```python
from build123d import *

# Parameters (mm, degrees)
MODEL_R                 = 1.5
SALIENTE_EXTRUIR1_DEPTH = 3


with BuildPart() as part:
    # Model → Saliente-Extruir1 (new body)
    with BuildSketch(Plane.XY):
        with BuildLine():
            Line((348.865624859, 201.955720999), (341.183644344, 209.637701515))
            ThreePointArc((341.183644344, 209.637701515), (334.819683313, 209.637701515), (334.819683313, 203.273740484))
            Line((334.819683313, 203.273740484), (343.819683313, 194.273740484))
            ThreePointArc((343.819683313, 194.273740484), (344.50159778, 193.714107744), (345.279588383, 193.298263103))
            Line((345.279588383, 193.298263103), (372.279588383, 175.298263103))
            ThreePointArc((372.279588383, 175.298263103), (373.123757379, 175.042187237), (374.001663828, 174.955720999))
            Line((374.001663828, 174.955720999), (383.001663828, 174.955720999))
            ThreePointArc((383.001663828, 174.955720999), (387.501663828, 179.455720999), (383.001663828, 183.955720999))
            Line((383.001663828, 183.955720999), (375.865624859, 183.955720999))
            Line((375.865624859, 183.955720999), (369.501663828, 190.31968203))
            Line((369.501663828, 190.31968203), (369.501663828, 197.455720999))
            ThreePointArc((369.501663828, 197.455720999), (368.183644344, 200.637701515), (365.001663828, 201.955720999))
            Line((365.001663828, 201.955720999), (348.865624859, 201.955720999))
        make_face()
        with Locations((347.001663829, 197.455720999)):
            Circle(MODEL_R, mode=Mode.SUBTRACT)
        with Locations((338.001663828, 206.455720999)):
            Circle(MODEL_R, mode=Mode.SUBTRACT)
        with Locations((365.001663828, 188.455720999)):
            Circle(MODEL_R, mode=Mode.SUBTRACT)
        with Locations((356.001663828, 197.455720999)):
            Circle(MODEL_R, mode=Mode.SUBTRACT)
        with Locations((383.001663828, 179.455720999)):
            Circle(MODEL_R, mode=Mode.SUBTRACT)
        with Locations((365.001663828, 197.455720999)):
            Circle(MODEL_R, mode=Mode.SUBTRACT)
    extrude(amount=SALIENTE_EXTRUIR1_DEPTH)


solid = part.part
```
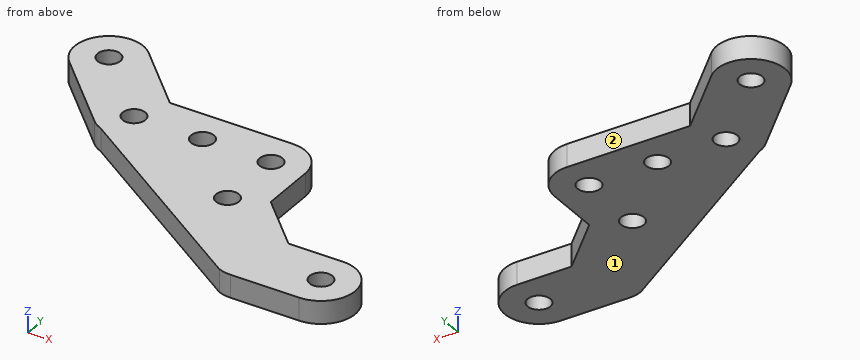
The model under review builds one solid part; all positions refer to its coordinate system, in mm. Face numbers are marked on the shaded views. A direction names the side the tool comes from. Coordinates: 2 decimals unless noted, no trailing zeros. Order: outer loops, then holes, each group sorted by start corner. A loop starts at its lowest first (then second) coordinate and runs counter-clockwise, first axis right, second up. Notation, with made-up numbers: (63.5, 47.5) -> (114.5, 47.5) arc R19 ccw to (114.5, 65.5) -> close; hole circle Ø9 at (-31.5, 51). An arc over 180 degrees is marked (long way). Answer in a Markdown table with one row per item. Add a question column.
Item 1: Clearance check with flat-ended pins moving along their axes: pin 1 (0.9 mm diameter, centred on y = 193, z = 1, fed in from +X); pin 2 (1.5 mm diameter, centred on x = 368, z = 1, fed in from -Y); pin 3 (0.9 mm diameter, centred on x = 358.5, z = 2, fed in from +Y). State where each tip first meets the part, or that it passes through.
Item 2: To check wall thickness, follow probe 1 along X at (y, z) = (198, 1.7); probe 2 along Y at (x, z) = (376.5, 1.7); probe 3 along Y at (x, z) = (355, 0.85). State the ranges of each line that lie inside material, in increasing order.
Item 3: We need section C-C on z = 0.5. Write out the cut boundary in (x, y).
Item 4: We need section D-D on x = 380.5. Write out the cut boundary in (y, z), plus the area to 3 significant figures.
Item 5: Machinability: for the marked faces 1 and 2, which of the approach directions +Z, -Z, +X, -X, +Y, -Y give a long, thin tool a straight path to every point of the face, cutting with its end or side? Answer none if there is none.
Item 6: We need section B-B on x = 347.5. Write out the cut boundary in (y, z).
Item 7: We need section A-A on y = 205.5. Write out the cut boundary in (x, z).
Final values:
| question | item | result |
|---|---|---|
| 1 | pin 1 | stops at x = 369.5 |
| 1 | pin 2 | stops at y = 177.65 |
| 1 | pin 3 | stops at y = 201.96 |
| 2 | probe 1 | x = 340.09 to 345.6, 348.4 to 354.6, 357.4 to 363.6, 366.4 to 369.47 |
| 2 | probe 2 | y = 174.96 to 183.96 |
| 2 | probe 3 | y = 186.82 to 196.34, 198.57 to 201.96 |
| 3 | outline | (334.82, 203.27) -> (343.82, 194.27) arc R4.5 ccw to (345.28, 193.3) -> (372.28, 175.3) arc R4.5 ccw to (374, 174.96) -> (383, 174.96) arc R4.5 ccw to (383, 183.96) -> (375.87, 183.96) -> (369.5, 190.32) -> (369.5, 197.46) arc R4.5 ccw to (365, 201.96) -> (348.87, 201.96) -> (341.18, 209.64) arc R4.5 ccw to start; hole circle Ø3 at (338, 206.46); hole circle Ø3 at (347, 197.46); hole circle Ø3 at (356, 197.46); hole circle Ø3 at (365, 188.46); hole circle Ø3 at (365, 197.46); hole circle Ø3 at (383, 179.46) |
| 4 | outline | (174.96, 0) -> (183.96, 0) -> (183.96, 3) -> (174.96, 3) -> close |
| 4 | area | 27.0 mm2 |
| 5 | face 1 | -Z, +X, -X, +Y, -Y |
| 5 | face 2 | +Z, -Z, +X, +Y |
| 6 | outline | (191.82, 0) -> (196.04, 0) -> (196.04, 3) -> (191.82, 3) -> close; (198.87, 0) -> (203.32, 0) -> (203.32, 3) -> (198.87, 3) -> close |
| 7 | outline | (333.6, 0) -> (336.85, 0) -> (336.85, 3) -> (333.6, 3) -> close; (339.16, 0) -> (345.32, 0) -> (345.32, 3) -> (339.16, 3) -> close |
